Work out the finished part from the listing and answer in its coordinate system (mm). A direction names the side the tool comes from. Coordinates: 2 decimals unless noted, no trailing zeros. Loops run counter-clockwise (first coordinate to the right, second up) from the corner with the lowest first, then second, coordinate; pieces in that order, holes last. Notation, with made-up numbers: (-32, 71.25) - (-4, 71.25) arc R17 cw to (-4, 98.25) - close; hole circle Ø8 at (-33, 68.5). An arc over 180 degrees is marked (long way). Write each question's results on one line, items separated by ' | '. Start each with the question number.
1. A cutting plane is placed at A-A on x = 0. Determine the outline of the cut face in (y, z).
2. Find the intervals of material crossed by line 1 along Y through (x, z) = (0, 1.45); line 2 along Y through (x, z) = (50, 4.6); line 3 along Y through (x, z) = (12, 2.4), in increasing order. Write a range as [from, to].
3. A cutting plane is placed at B-B on y = 0. State how many separate pieces and enclosed holes the cut face has, then the cut area to 3 significant figures.
4. Which of the six approach directions +Z, -Z, +X, -X, +Y, -Y give full straight-line access (tool end or side, diameter ignored) to faces 1 (the cylindrical face through (51.847, -0.766, 4.396)), 2 (the flat face through (25, 2, 2)), 3 (the cylindrical face through (46.93, -2.19, 2.37))?
5. This flat-tipped pin is pushed along its axis until it touches: P1, Ø2.5, axis at x = 27, z = 3, coming from the +Y side. Where does it stop, or does it pass through?
6. A cutting plane is placed at C-C on x = 38.5. Determine the outline of the cut face in (y, z), then the cut area to 3 significant figures.
7. Determine the mould class of faces 4 (the flat face through (25, 0, 4.8)), 5 (the flat face through (25, -2, 2)) for opening direction X: released by +X, released by -X, zero draft, split by the parting line, or undercut.
from build123d import *

# Parameters (mm, degrees)
SKETCH1_R           = 1.2
BOSS_EXTRUDE1_DEPTH = 4.8
SKETCH2_R           = 2
CUT_EXTRUDE1_DEPTH  = 1.8
FILLET1_R           = 1


with BuildPart() as part:
    # Sketch1 → Boss-Extrude1 (new body)
    with BuildSketch(Plane.XY):
        with BuildLine():
            Line((5, -2), (45, -2))
            ThreePointArc((45, -2), (46.961161351, -2.194193243), (48.846153846, -2.769230769))
            ThreePointArc((48.846153846, -2.769230769), (53, 0), (48.846153846, 2.769230769))
            ThreePointArc((48.846153846, 2.769230769), (46.961161351, 2.194193243), (45, 2))
            Line((45, 2), (5, 2))
            ThreePointArc((5, 2), (3.038838649, 2.194193243), (1.153846154, 2.769230769))
            ThreePointArc((1.153846154, 2.769230769), (-3, 0), (1.153846154, -2.769230769))
            ThreePointArc((1.153846154, -2.769230769), (3.038838649, -2.194193243), (5, -2))
        make_face()
        Circle(SKETCH1_R, mode=Mode.SUBTRACT)
        with Locations((50, 0)):
            Circle(SKETCH1_R, mode=Mode.SUBTRACT)
    extrude(amount=BOSS_EXTRUDE1_DEPTH)

    # Sketch2 → Cut-Extrude1 (cut)
    with BuildSketch(Plane.XY.offset(4.8)):
        with Locations((50, 0)):
            Circle(SKETCH2_R)
    extrude(amount=-CUT_EXTRUDE1_DEPTH, mode=Mode.SUBTRACT)

    # Fillet1
    # the kernel refuses this fillet: 1 mm, written as the material it adds along each edge
    with BuildSketch(Plane(origin=(50, 0, 3), x_dir=(1, 0, 0), z_dir=(0, -1, 0))) as fillet1_piece_1:
        with BuildLine():
            CenterArc((1, 0.979795897), FILLET1_R, 281.536959033, 78.463040967)
            Line((1.2, 0), (1.204, -0.019595918))
            ThreePointArc((1.204, -0.019595918), (1.6, -0.02), (2, -0.02))
            Line((2, -0.02), (2.02, 0))
            Line((2.02, 0), (2.02, 0.979795897))
            Line((2.02, 0.979795897), (2, 0.979795897))
        make_face()
    revolve(axis=Axis((50, 0, 3), (0, 0, 1)))


solid = part.part
Values:
1) outline: (-3, 0) - (-1.2, 0) - (-1.2, 4.8) - (-3, 4.8) - close; (1.2, 0) - (3, 0) - (3, 4.8) - (1.2, 4.8) - close
2) line 1: [-3, -1.2], [1.2, 3] | line 2: [-3, -2], [2, 3] | line 3: [-2, 2]
3) separate pieces: 3 | enclosed holes: 0 | area: 243 mm^2
4) face 1: +Z | face 2: +Z, -Z, +Y | face 3: +Z, -Z, -Y
5) P1: y = 2
6) outline: (-2, 0) - (2, 0) - (2, 4.8) - (-2, 4.8) - close | area: 19.2 mm^2
7) face 4: zero draft | face 5: undercut
